Source: CAD feature listing. Evaluate the final solid. Frame: model axes, mm. Coordinates: 2 decimals unless noted, no trailing zeros. Loops run counter-clockwise (first coordinate to the right, second up) from the corner with the lowest first, then second, coordinate; pieces in that order, holes last.
from build123d import *

# Parameters (mm, degrees)
BOSS_EXTRUDE1_DEPTH = 1.5875


with BuildPart() as part:
    # Sketch1 → Boss-Extrude1 (new body, symmetric)
    with BuildSketch(Plane.XY):
        Polygon((-150.011928505, -117.303446964), (-7.136928505, -117.303446964), (-7.136928505, -72.853446964), (-35.711928505, -53.803446964), (-150.011928505, -53.803446964), align=None)
    extrude(amount=BOSS_EXTRUDE1_DEPTH, both=True)


solid = part.part
Q1. Section B-B, the plane y = -66. Return the cut outline in (x, z).
Q2. Section A-A, the plane z = 0.5. Return the cut outline in (x, y), plus the area to 3 significant figures.
Q3. Section C-C, the plane x = -19.5. Return the cut outline in (y, z).
Q4. Line query: line 1 along Y through (x, z) = (-17, -1.15); line 2 along Y through (x, z) = (-22.5, 0.8); line 3 along X through (y, z) = (-63.5, -1.35). Output: solid intervals per line, ascending.
Derived:
1. outline: (-150.01, -1.59) - (-17.42, -1.59) - (-17.42, 1.59) - (-150.01, 1.59) - close
2. outline: (-150.01, -117.3) - (-7.14, -117.3) - (-7.14, -72.85) - (-35.71, -53.8) - (-150.01, -53.8) - close
2. area: 8,800 mm2
3. outline: (-117.3, -1.59) - (-64.61, -1.59) - (-64.61, 1.59) - (-117.3, 1.59) - close
4. line 1: y = -117.3 to -66.28
4. line 2: y = -117.3 to -62.61
4. line 3: x = -150.01 to -21.17
